```python
from build123d import *

# Parameters (mm, degrees)
F1_DEPTH = 40.2336
F0_R     = 10.16
F2_DEPTH = 15.7734
F3_R     = 3.302


with BuildPart() as f1:
    # F0 (on Top) → F1 (new body)
    with BuildSketch(Plane.XY):
        with BuildLine():
            ThreePointArc((5.211817, -28.095686), (21.971098, -18.270235), (28.575, 0))
            ThreePointArc((28.575, 0), (21.971098, 18.270235), (5.211817, 28.095686))
            ThreePointArc((5.211817, 28.095686), (-28.575, 0), (5.211817, -28.095686))
        make_face()
        with BuildLine():
            ThreePointArc((-13.447765, 4.826), (0, 14.2875), (13.447765, 4.826))
            Line((13.447765, 4.826), (18.5293, 4.826))
            Line((18.5293, 4.826), (18.5293, -4.826))
            Line((18.5293, -4.826), (13.447765, -4.826))
            ThreePointArc((13.447765, -4.826), (0, -14.2875), (-13.447765, -4.826))
            Line((-13.447765, -4.826), (-18.5293, -4.826))
            Line((-18.5293, -4.826), (-18.5293, 4.826))
            Line((-18.5293, 4.826), (-13.447765, 4.826))
        make_face(mode=Mode.SUBTRACT)
        with BuildLine():
            ThreePointArc((-13.447765, -4.826), (-14.2875, 0), (-13.447765, 4.826))
            Line((-13.447765, 4.826), (-18.5293, 4.826))
            Line((-18.5293, 4.826), (-18.5293, -4.826))
            Line((-18.5293, -4.826), (-13.447765, -4.826))
        make_face()
    extrude(amount=F1_DEPTH)

    # F0 (on Top) → F2 (join)
    with BuildSketch(Plane.XY):
        with BuildLine():
            ThreePointArc((5.211817, -28.095686), (21.971098, -18.270235), (28.575, 0))
            ThreePointArc((28.575, 0), (21.971098, 18.270235), (5.211817, 28.095686))
            ThreePointArc((5.211817, 28.095686), (-28.575, 0), (5.211817, -28.095686))
        make_face()
        with BuildLine():
            ThreePointArc((-13.447765, 4.826), (0, 14.2875), (13.447765, 4.826))
            Line((13.447765, 4.826), (18.5293, 4.826))
            Line((18.5293, 4.826), (18.5293, -4.826))
            Line((18.5293, -4.826), (13.447765, -4.826))
            ThreePointArc((13.447765, -4.826), (0, -14.2875), (-13.447765, -4.826))
            Line((-13.447765, -4.826), (-18.5293, -4.826))
            Line((-18.5293, -4.826), (-18.5293, 4.826))
            Line((-18.5293, 4.826), (-13.447765, 4.826))
        make_face(mode=Mode.SUBTRACT)
        with BuildLine():
            ThreePointArc((5.211817, 28.095686), (21.971098, 18.270235), (28.575, 0))
            ThreePointArc((28.575, 0), (21.971098, -18.270235), (5.211817, -28.095686))
            Line((5.211817, -28.095686), (53.975, -19.05))
            ThreePointArc((53.975, -19.05), (73.025, 0), (53.975, 19.05))
            Line((53.975, 19.05), (5.211817, 28.095686))
        make_face()
        with Locations((53.975, 0)):
            Circle(F0_R, mode=Mode.SUBTRACT)
    extrude(amount=F2_DEPTH)

    # F3
    f3_edges = [f1.edges().sort_by_distance(p)[0] for p in [
        (-5.211817, 28.095686, 40.2336),
    ]]
    fillet(f3_edges, radius=F3_R)


solid = f1.part
```
Geometry check sheet. Reference: the model listing, model coordinates, mm. A direction names the side the tool comes from. Round coordinates to 2 decimals unless told otherwise and drop trailing zeros. Return JSON: item names as keys, results as strings. Group by question number.
Q1. Gauge pin test, flat ends, axial feed: pin 1 (5 mm diameter, centred on x = 50.5, z = 7, fed in from -Y); pin 2 (5.5 mm diameter, centred on x = 16.5, z = 24.5, fed in from -Y); pin 3 (8 mm diameter, centred on x = 43, y = -7.5, fed in from +Z). Record the tip position at first contact, or that the pin passes through.
Q2. Section check B-B, the plane z = 3.5. Count the separate pieces of the cut face and the enclosed holes in it, plus the area to 3 significant figures.
Q3. Release check for a two-part mould opening along Y. For faces 1 (the flat face through (39, 0, 15.773)), 2 (the flat face through (16, -4.826, 20)), 3 (the flat face through (29.252, -23.636, 7.776)) record: released by +Y, released by -Y, zero draft, split by the parting line, or undercut.
Q4. Material ranges on probe 1 along Z at (x, y) = (30.5, 13.5); probe 2 along X at (y, z) = (-6, 22.5); probe 3 along X at (y, z) = (-10.5, 18), recorded low to high. Write a range as from..to.
Q5. Tool access check on faces 4 (the flat face through (22, 0, 0)), 5 (the flat face through (16, 4.826, 20)). Record the directions out of +Z, -Z, +X, -X, +Y, -Y that give a thin tool (end or side, any length) a straight path to the whole face; none if there is none.
Numbers:
{
 "1": {"pin 1": "y = -20.16", "pin 2": "y = -25.05", "pin 3": "z = 15.77"},
 "2": {"separate pieces": "1", "enclosed holes": "2", "area": "3,440 mm^2"},
 "3": {"face 1": "zero draft", "face 2": "undercut", "face 3": "released by -Y"},
 "4": {"probe 1": "0..15.77", "probe 2": "-27.94..-12.97, 12.97..27.94", "probe 3": "-26.58..-9.69, 9.69..26.58"},
 "5": {"face 4": "-Z, +X, -X, +Y, -Y", "face 5": "+Z, -Z"}
}
